```python
from build123d import *

# Parameters (mm, degrees)
SKETCH1_R         = 11.9126
SHAFT_DEPTH       = 6.6802
SKETCH4_R         = 11.938
CAP_DEPTH         = 1.524
SKETCH7_R         = 8.89
TOP_HOLE_DEPTH    = 2.286
SKETCH8_R         = 9.6647
BOTTOM_HOLE_DEPTH = 18.445362755
DRAFT1_ANGLE      = 0.25
SKETCH9_R         = 0.635
SIDE_HOLES_DEPTH  = 1.524


with BuildPart() as part:
    # Sketch1 → Shaft (new body)
    with BuildSketch(Plane(origin=(0, 0, 0), x_dir=(1, 0, 0), z_dir=(0, 1, 0))):
        with Locations(Location((0, 0, 0), (0, 0, 270))):
            Circle(SKETCH1_R)
    extrude(amount=-SHAFT_DEPTH)

    # Sketch4 → Cap (add)
    with BuildSketch(Plane(origin=(0, 0, 0), x_dir=(-1, 0, 0), z_dir=(0, 1, 0))):
        with Locations(Location((0, 0, 0), (0, 0, 90))):
            Circle(SKETCH4_R)
    extrude(amount=-CAP_DEPTH)

    # Sketch7 → Top Hole (cut)
    with BuildSketch(Plane(origin=(0, 0, 0), x_dir=(-1, 0, 0), z_dir=(0, 1, 0))):
        with Locations(Location((0, 0, 0), (0, 0, 90))):
            Circle(SKETCH7_R)
    extrude(amount=-TOP_HOLE_DEPTH, mode=Mode.SUBTRACT)

    # Sketch8 → Bottom Hole (cut, through all)
    with BuildSketch(Plane(origin=(0, -2.286, 0), x_dir=(-1, 0, 0), z_dir=(0, 1, 0))):
        with Locations(Location((0, 0, 0), (0, 0, 90))):
            Circle(SKETCH8_R)
    extrude(amount=-BOTTOM_HOLE_DEPTH, mode=Mode.SUBTRACT)

    # Draft1
    draft1_faces = [part.faces().sort_by_distance(p)[0] for p in [
        (0, -4.4831, -9.6647),
    ]]
    draft(draft1_faces, Plane(origin=(0, -6.6802, 0), x_dir=(0, 0, -1), z_dir=(0, -1, 0)), DRAFT1_ANGLE)

    # Sketch9 → Side Holes (cut)
    with BuildSketch(Plane(origin=(0, 0, 0), x_dir=(-1, 0, 0), z_dir=(0, 1, 0))):
        with Locations(Location((0, -10.414, 0), (0, 0, 90))):
            Circle(SKETCH9_R)
        with Locations(Location((0, 10.414, 0), (0, 0, 270))):
            Circle(SKETCH9_R)
    extrude(amount=-SIDE_HOLES_DEPTH, mode=Mode.SUBTRACT)


solid = part.part
```
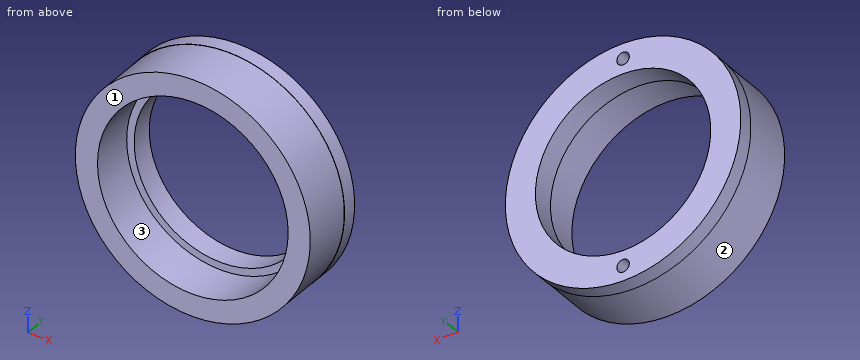
For this review, take the finished solid that the model builds, in its own axes (mm). Face numbers are marked on the shaded views. Round coordinates to 2 decimals unless told otherwise and drop trailing zeros. Order: outer loops, then holes, each group sorted by start corner. A loop starts at its lowest first (then second) coordinate and runs counter-clockwise, first axis right, second up. Notation, with made-up numbers: (-20, 84) -> (35, 84) arc R23 cw to (35, 93) -> close; hole circle Ø5 at (77.5, 13). An arc over 180 degrees is marked (long way). Use a Markdown table: item, result.
Item 1: For line 1 along X through (y, z) = (-1.75, 0); line 2 along Z through (x, y) = (-0.25, -6.5); line 3 along Z through (x, y) = (-2.25, -3.25), list the stretches that pass through material, from the lowest coordinate up. Write a range as [from, to].
Resolved:
| item | result |
|---|---|
| line 1 | x = [-11.91, -8.89], [8.89, 11.91] |
| line 2 | z = [-11.91, -9.66], [9.66, 11.91] |
| line 3 | z = [-11.7, -9.38], [9.38, 11.7] |
Item 2: Take a section at A-A (y = -2). State the section outline as (x, z) points, plus the area to 3 significant figures.
Resolved:
| item | result |
|---|---|
| outline | circle Ø23.83 at (0, 0); hole circle Ø17.78 at (0, 0) |
| area | 198 mm² |
Item 3: For pin 1 (1.5 mm diameter, centred on x = 6, y = -3.5, fed in from +Z); pin 2 (0.6 mm diameter, centred on x = 0, z = 10.5, fed in from +Y); pin 3 (2 mm diameter, centred on x = 1.5, y = -4, fed in from -Z), all flat-tipped, find the tip position at first contact; note any pin that passes through.
Resolved:
| item | result |
|---|---|
| pin 1 | stops at z = 10.69 |
| pin 2 | stops at y = -1.52 |
| pin 3 | stops at z = -11.9 |
Item 4: Take a section at B-B (y = -4.25). State the section outline as (x, z) points, plus the area to 3 significant figures.
Resolved:
| item | result |
|---|---|
| outline | circle Ø23.83 at (0, 0); hole circle Ø19.31 at (0, 0) |
| area | 153 mm² |
Item 5: Draft analysis for pull direction Z (two halves, no side actions). For the marked faces 1, 2 and 3, state which applies: +Z half, -Z half, draft (parallel to the pull), parting line (faces both ways), or undercut.
Resolved:
| item | result |
|---|---|
| face 1 | draft |
| face 2 | parting line |
| face 3 | undercut |
